The model under review builds one solid part; all positions refer to its coordinate system, in mm. Face numbers are marked on the shaded views. A direction names the side the tool comes from. Give positions to 0.01 mm unless a question says otherwise; leave off trailing zeros. Loops run counter-clockwise (first coordinate to the right, second up) from the corner with the lowest first, then second, coordinate; pieces in that order, holes last. Notation, with made-up numbers: M 3.25,-9 L 41.25,-9 A24 cw 41.25,17 Z; hole C 9.5,4 d4. An arc over 180 degrees is marked long. Return JSON: item names as keys, results as strings. Group by question number.
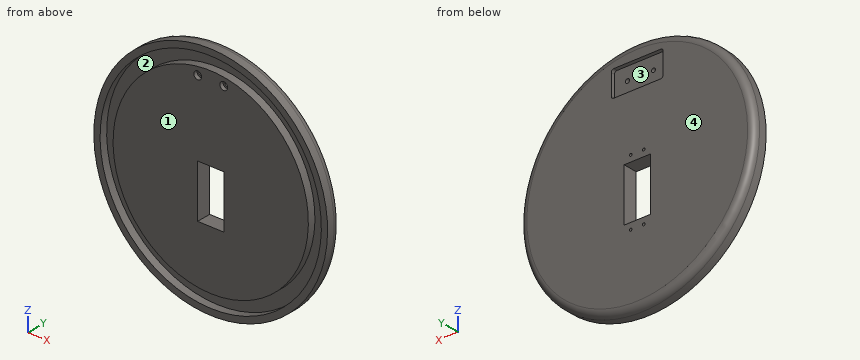
```python
from build123d import *

# Parameters (mm, degrees)
SKETCH1_R           = 90
BOSS_EXTRUDE1_DEPTH = 11
SKETCH7_W           = 40
SKETCH7_H           = 20
CUT_EXTRUDE7_DEPTH  = 3
SKETCH12_R          = 1.55
CUT_EXTRUDE8_DEPTH  = 20
SKETCH13_R          = 3
CUT_EXTRUDE9_DEPTH  = 3
FILLET1_R           = 2
FILLET2_R           = 2
FILLET3_R           = 2
FILLET4_R           = 2
SKETCH15_R          = 85.2
SKETCH15_R_2        = 75.2
CUT_EXTRUDE10_DEPTH = 6
FILLET5_R           = 5
SKETCH16_W          = 20.139846291
SKETCH16_H          = 40.720332108
CUT_EXTRUDE13_DEPTH = 20
SKETCH17_R          = 1
CUT_EXTRUDE14_DEPTH = 10


with BuildPart() as part:
    # Sketch1 → Boss-Extrude1 (new body)
    with BuildSketch(Plane(origin=(0, 0, 0), x_dir=(1, 0, 0), z_dir=(0, 1, 0))):
        with Locations(Location((0, 0, 0), (0, 0, 270))):
            Circle(SKETCH1_R)
    extrude(amount=BOSS_EXTRUDE1_DEPTH)

    # Sketch7 → Cut-Extrude7 (cut)
    with BuildSketch(Plane(origin=(0, 11, 0), x_dir=(1, 0, 0), z_dir=(0, 1, 0))):
        with Locations((0, -68.46128741)):
            Rectangle(SKETCH7_W, SKETCH7_H)
    extrude(amount=-CUT_EXTRUDE7_DEPTH, mode=Mode.SUBTRACT)

    # Sketch12 → Cut-Extrude8 (cut)
    with BuildSketch(Plane(origin=(0, 8, 0), x_dir=(1, 0, 0), z_dir=(0, 1, 0))):
        with Locations(Location((10, -68.46128741, 0), (0, 0, 270))):
            Circle(SKETCH12_R)
        with Locations(Location((-10, -68.46128741, 0), (0, 0, 270))):
            Circle(SKETCH12_R)
    extrude(amount=-CUT_EXTRUDE8_DEPTH, mode=Mode.SUBTRACT)

    # Sketch13 → Cut-Extrude9 (cut)
    with BuildSketch(Plane.XZ):
        with Locations(Location((10, 68.46128741, 0), (0, 0, 270))):
            Circle(SKETCH13_R)
        with Locations(Location((-10, 68.46128741, 0), (0, 0, 270))):
            Circle(SKETCH13_R)
    extrude(amount=-CUT_EXTRUDE9_DEPTH, mode=Mode.SUBTRACT)

    # Fillet1
    fillet1_edges = [part.edges().sort_by_distance(p)[0] for p in [
        (-20, 9.5, 58.46128741),
    ]]
    fillet(fillet1_edges, radius=FILLET1_R)

    # Fillet2
    fillet2_edges = [part.edges().sort_by_distance(p)[0] for p in [
        (20, 9.5, 58.46128741),
    ]]
    fillet(fillet2_edges, radius=FILLET2_R)

    # Fillet3
    fillet3_edges = [part.edges().sort_by_distance(p)[0] for p in [
        (-20, 9.5, 78.46128741),
    ]]
    fillet(fillet3_edges, radius=FILLET3_R)

    # Fillet4
    fillet4_edges = [part.edges().sort_by_distance(p)[0] for p in [
        (20, 9.5, 78.46128741),
    ]]
    fillet(fillet4_edges, radius=FILLET4_R)

    # Sketch15 → Cut-Extrude10 (cut)
    with BuildSketch(Plane.XZ):
        with Locations(Location((0, 0, 0), (0, 0, 270))):
            Circle(SKETCH15_R)
        with Locations(Location((0, 0, 0), (0, 0, 270))):
            Circle(SKETCH15_R_2, mode=Mode.SUBTRACT)
    extrude(amount=-CUT_EXTRUDE10_DEPTH, mode=Mode.SUBTRACT)

    # Fillet5
    fillet5_edges = [part.edges().sort_by_distance(p)[0] for p in [
        (0, 11, -90),
    ]]
    fillet(fillet5_edges, radius=FILLET5_R)

    # Sketch16 → Cut-Extrude13 (cut)
    with BuildSketch(Plane(origin=(0, 11, 0), x_dir=(1, 0, 0), z_dir=(0, 1, 0))):
        with Locations((0.000598288, 9.704977579)):
            Rectangle(SKETCH16_W, SKETCH16_H)
    extrude(amount=-CUT_EXTRUDE13_DEPTH, mode=Mode.SUBTRACT)

    # Sketch17 → Cut-Extrude14 (cut)
    with BuildSketch(Plane(origin=(0, 11, 0), x_dir=(1, 0, 0), z_dir=(0, 1, 0))):
        with Locations(Location((-5, 34.9655003, 0), (0, 0, 270))):
            Circle(SKETCH17_R)
        with Locations(Location((5, 34.9655003, 0), (0, 0, 270))):
            Circle(SKETCH17_R)
        with Locations(Location((-5, -15.5345003, 0), (0, 0, 270))):
            Circle(SKETCH17_R)
        with Locations(Location((5, -15.5345003, 0), (0, 0, 270))):
            Circle(SKETCH17_R)
    extrude(amount=-CUT_EXTRUDE14_DEPTH, mode=Mode.SUBTRACT)


solid = part.part
```
(1) Mouldability with a two-part tool opening along X and no side actions: class the marked faces 1 and 2 as released by +X, released by -X, zero draft, split by the parting line, or undercut.
(2) For probe 1 along X at (y, z) = (1.75, 5); probe 2 along X at (y, z) = (5.25, -49); probe 3 along Z at (x, y) = (38, 3.25), list the stretches that pass through material, from the lowest coordinate up.
(3) For the marked faces 3 and 4, list the 3-axis set-ups (+Z, -Z, +X, -X, +Y, -Y) from which the entire face can be reached by the end or side of a thin tool; tool diameter is ignored.
(4) Add section A-A (x = 0). Write out the cut boundary in (y, z).
(5) For pin 1 (10 mm diameter, centred on x = 9, z = 71.5, fed in from +Y); pin 2 (2 mm diameter, centred on x = 22.5, y = 6, fed in from +Z); pin 3 (5.5 mm diameter, centred on x = -3, y = 3.5, fed in from +Z); pin 4 (4 mm diameter, centred on x = 62, z = 18, fed in from -Y), all flat-tipped, find the tip position at first contact; note any pin that passes through.
Verdict:
{
 "1": {"face 1": "zero draft", "face 2": "undercut"},
 "2": {"probe 1": "x = -89.86 to -85.05, -75.03 to -10.07, 10.07 to 75.03, 85.05 to 89.86", "probe 2": "x = -75.49 to -69.7, -57.04 to 57.04, 69.7 to 75.49", "probe 3": "z = -81.58 to -76.26, -64.89 to 64.89, 76.26 to 81.58"},
 "3": {"face 3": "+Y", "face 4": "+Z, -Z, +X, -X, +Y"},
 "4": {"outline": "M 0,-90 L 6,-90 A5 ccw 11,-85 L 11,-30.07 L 0,-30.07 L 0,-75.2 L 6,-75.2 L 6,-85.2 L 0,-85.2 Z; M 0,10.66 L 11,10.66 L 11,58.46 L 8,58.46 L 8,78.46 L 11,78.46 L 11,85 A5 ccw 6,90 L 0,90 L 0,85.2 L 6,85.2 L 6,75.2 L 0,75.2 Z"},
 "5": {"pin 1": "stops at y = 8", "pin 2": "stops at z = 87.39", "pin 3": "stops at z = 90", "pin 4": "stops at y = 0"}
}
